Verification items for the finished model (mm, model axes). A direction names the side the tool comes from. Give positions to 0.01 mm unless a question says otherwise; leave off trailing zeros. Write each loop counter-clockwise with the first axis right and the second up, starting at its lowest first coordinate (ties: lowest second). Pieces come first, ordered by that corner, then holes. Notation, with made-up numbers: M 40.25,-17 L 75.25,-17 A24 cw 75.25,16 Z; hole C 19,72.25 d4. An arc over 180 degrees is marked long. Write item = value, one per line.
from build123d import *

# Parameters (mm, degrees)
BOSS_EXTRUDE1_DEPTH = 9.5
SKETCH2_R           = 2.25
CUT_EXTRUDE1_DEPTH  = 12
FILLET1_R           = 1


with BuildPart() as part:
    # Sketch1 → Boss-Extrude1 (new body)
    with BuildSketch(Plane(origin=(0, 0, 0), x_dir=(0, 0, -1), z_dir=(1, 0, 0))):
        Polygon((-7, 1.1), (7, 1.1), (7, -2.5), (13, -5.5), (18.5, -5.5), (18.5, 5.5), (-18.5, 5.5), (-18.5, -5.5), (-13, -5.5), (-7, -2.5), align=None)
    extrude(amount=BOSS_EXTRUDE1_DEPTH)

    # Sketch2 → Cut-Extrude1 (cut, through all)
    with BuildSketch(Plane(origin=(0, 5.5, 0), x_dir=(1, 0, 0), z_dir=(0, 1, 0))):
        with Locations((4.2, -12.75)):
            Circle(SKETCH2_R)
        with Locations((4.2, 12.75)):
            Circle(SKETCH2_R)
    extrude(amount=-CUT_EXTRUDE1_DEPTH, mode=Mode.SUBTRACT)

    # Fillet1
    fillet1_edges = [part.edges().sort_by_distance(p)[0] for p in [
        (4.75, 5.5, 18.5),
        (4.75, 5.5, -18.5),
        (4.75, -2.5, -7),
        (4.75, 1.1, -7),
        (4.75, 1.1, 7),
        (4.75, -2.5, 7),
    ]]
    fillet(fillet1_edges, radius=FILLET1_R)


solid = part.part
1) Draft check along Z on faces 3 (the cylindrical face through (4.816, 5.199, -18.215)), 4 (the cylindrical face through (4.816, 5.215, 18.199)), 5 (the cylindrical face through (4.816, 0.815, 6.699)), 6 (the flat face through (5, -1, 7)). Enter one of: +Z half, -Z half, draft (parallel to the pull), parting line (faces both ways), or undercut.
From the geometry:
face_3 = -Z half
face_4 = +Z half
face_5 = undercut
face_6 = undercut
2) Cross-section at B-B on x = 4.2. Record the boundary of the cut face in (y, z).
From the geometry:
outline = M -5.5,-18.5 L 4.5,-18.5 A1 ccw 5.5,-17.5 L 5.5,-15 L -5.5,-15 Z; M -5.5,15 L 5.5,15 L 5.5,17.5 A1 ccw 4.5,18.5 L -5.5,18.5 Z; M -4.25,-10.5 L 5.5,-10.5 L 5.5,10.5 L -4.25,10.5 L -2.78,7.55 A1 ccw -1.88,7 L 0.1,7 A1 cw 1.1,6 L 1.1,-6 A1 cw 0.1,-7 L -1.88,-7 A1 ccw -2.78,-7.55 Z
3) Material ranges on probe 1 along Z at (x, y) = (4.2, 1.75); probe 2 along Z at (x, y) = (4.2, -1.75); probe 3 along X at (y, z) = (0.25, 12.75), recorded low to high. Write a range as from..to.
From the geometry:
probe_1 = -18.5..-15, -10.5..10.5, 15..18.5
probe_2 = -18.5..-15, -10.5..-7, 7..10.5, 15..18.5
probe_3 = 0..1.95, 6.45..9.5
4) Cross-section at D-D on z = 11.5. Record the boundary of the cut face in (x, y), plus the area to 3 significant figures.
From the geometry:
outline = M 0,-4.75 L 2.33,-4.75 L 2.33,5.5 L 0,5.5 Z; M 6.07,-4.75 L 9.5,-4.75 L 9.5,5.5 L 6.07,5.5 Z
area = 59.0 mm^2
5) Cross-section at A-A on y = -3.5. Record the boundary of the cut face in (x, z).
From the geometry:
outline = M 0,-18.5 L 9.5,-18.5 L 9.5,-9 L 0,-9 Z; M 0,9 L 9.5,9 L 9.5,18.5 L 0,18.5 Z; hole C 4.2,-12.75 d4.5; hole C 4.2,12.75 d4.5
6) Depth check by flat-ended pin: P1, Ø4, axis at x = 4.2, z = -12.75, coming from the -Y side (3 decimals); P2, Ø3, axis at x = 4, z = 2, coming from the -Y side; P3, Ø1.5, axis at y = 3, z = 2.5, coming from the -X side. Enter the tip coordinate at first touch or a pass-through.
From the geometry:
P1 = through
P2 = 1.1
P3 = 0
7) Cross-section at C-C on y = 3.75. Record the boundary of the cut face in (x, z).
From the geometry:
outline = M 0,-18.5 L 9.5,-18.5 L 9.5,18.5 L 0,18.5 Z; hole C 4.2,-12.75 d4.5; hole C 4.2,12.75 d4.5
8) Tool access check on faces 1 (the flat face through (5, -1, -7)), 2 (the flat face through (5, -5.5, 16)). Record the directions out of +Z, -Z, +X, -X, +Y, -Y that give a thin tool (end or side, any length) a straight path to the whole face; none if there is none.
From the geometry:
face_1 = +X, -X, -Y
face_2 = +Z, -Z, +X, -X, -Y
